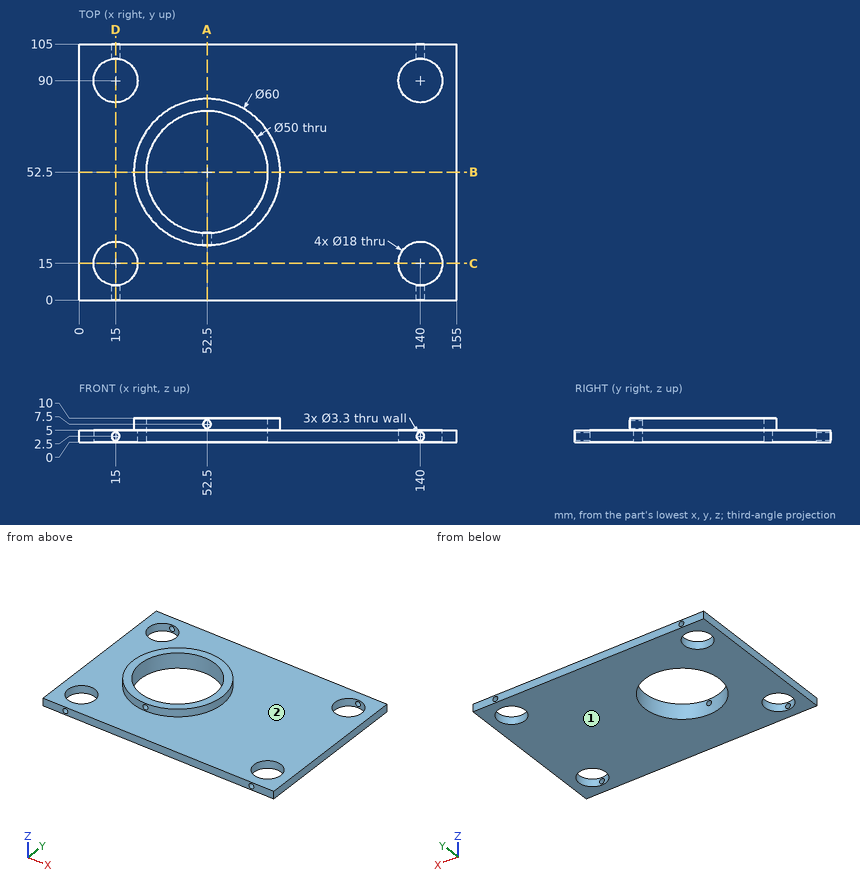
Study the drawing (mm; zero at the part's minimum x, y, z) and answer. A direction names the side the tool comes from. Round coordinates to 2 decimals unless told otherwise and drop trailing zeros. Write each loop counter-clockwise with the first axis right and the second up, starting at its lowest first coordinate (ties: lowest second). Pieces come first, ordered by that corner, then holes. Notation, with made-up numbers: (33, -22.5) -> (38, -22.5) arc R23 cw to (38, 15.5) -> close; hole circle Ø7 at (-6, 69). An arc over 180 degrees is marked (long way). Use CSV: the item, a comma, the result in double quotes. Start each with the question number.
(1) Each of these flat-tipped pins is pushed along its axis until it touches: pin 1 (11 mm diameter, centred on x = 15, y = 15, fed in from +Z); pin 2 (12 mm diameter, centred on x = 96, y = 28, fed in from +Z); pin 3 (3 mm diameter, centred on x = 140, z = 2.5, fed in from +Y); pin 4 (4 mm diameter, centred on x = 52.5, z = 7.5, fed in from +Y). Where does it stop, or does it pass through?
(2) Section C-C on y = 15 is taken. Give the vertices of the cut face in (x, z).
(3) Consider L1, parallel to Z at x = 140, y = 103.75; L2, parallel to X at y = 7, z = 3.25; L3, parallel to Y at x = 11.5, z = 4.5. Determine where each line is inside the solid, lowest interval first. Write a range as from..to.
(4) Section A-A on x = 52.5 is taken. Give the vertices of the cut face in (y, z), then the cut area to 4 significant figures.
(5) Section D-D on x = 15 is taken. Give the vertices of the cut face in (y, z).
(6) Which of the six approach directions +Z, -Z, +X, -X, +Y, -Y give full straight-line access (tool end or side, diameter ignored) to the marked faces 1 and 2?
(7) Section B-B on y = 52.5 is taken. Give the vertices of the cut face in (x, z), then the cut area to 3 significant figures.
A:
1,pin 1,"passes through"
1,pin 2,"stops at z = 5"
1,pin 3,"stops at y = 81.13"
1,pin 4,"stops at y = 82.5"
2,outline,"(0, 0) -> (6, 0) -> (6, 5) -> (0, 5) -> close; (24, 0) -> (131, 0) -> (131, 5) -> (24, 5) -> close; (149, 0) -> (155, 0) -> (155, 5) -> (149, 5) -> close"
3,L1,"z = 0..0.85, 4.15..5"
3,L2,"x = 0..10.88, 19.12..135.88, 144.12..155"
3,L3,"y = 0..6.71, 23.29..81.71, 98.29..105"
4,outline,"(0, 0) -> (27.5, 0) -> (27.5, 5.85) -> (22.5, 5.85) -> (22.5, 5) -> (0, 5) -> close; (22.5, 9.15) -> (27.5, 9.15) -> (27.5, 10) -> (22.5, 10) -> close; (77.5, 0) -> (105, 0) -> (105, 5) -> (82.5, 5) -> (82.5, 10) -> (77.5, 10) -> close"
4,area,"308.5 mm²"
5,outline,"(0, 0) -> (6, 0) -> (6, 0.85) -> (0, 0.85) -> close; (0, 4.15) -> (6, 4.15) -> (6, 5) -> (0, 5) -> close; (24, 0) -> (81, 0) -> (81, 5) -> (24, 5) -> close; (99, 0) -> (105, 0) -> (105, 0.85) -> (99, 0.85) -> close; (99, 4.15) -> (105, 4.15) -> (105, 5) -> (99, 5) -> close"
6,face 1,"-Z, +X, -X, +Y, -Y"
6,face 2,"+Z"
7,outline,"(0, 0) -> (27.5, 0) -> (27.5, 10) -> (22.5, 10) -> (22.5, 5) -> (0, 5) -> close; (77.5, 0) -> (155, 0) -> (155, 5) -> (82.5, 5) -> (82.5, 10) -> (77.5, 10) -> close"
7,area,"575 mm²"
